```python
from build123d import *

# Parameters (mm, degrees)
BOSS_EXTRUDE1_DEPTH       = 50.8
SHELL1_T                  = -6.35
FILLET1_R                 = 3.175
CUT_EXTRUDE1_DEPTH        = 2.54
F_2_64_TAPPED_HOLE1_D     = 1.778
F_2_64_TAPPED_HOLE1_DEPTH = 6.35
F_2_64_TAPPED_HOLE1_TIP   = 0.53416509


with BuildPart() as part:
    # Sketch2 → Boss-Extrude1 (new body)
    with BuildSketch(Plane(origin=(0, 0, 0), x_dir=(1, 0, 0), z_dir=(0, 1, 0))):
        with BuildLine():
            Line((0, 0), (139.7, 0))
            Line((139.7, 0), (139.7, 63.5))
            ThreePointArc((139.7, 63.5), (111.582381507, 95.881856359), (70.429678072, 107.95))
            Line((70.429678072, 107.95), (0, 107.95))
            Line((0, 107.95), (0, 0))
        make_face()
    extrude(amount=BOSS_EXTRUDE1_DEPTH)

    # Shell1
    shell1_openings = [part.faces().sort_by_distance(p)[0] for p in [
        (71.269444109, 50.8, -57.911371272),
    ]]
    offset(amount=SHELL1_T, openings=shell1_openings, kind=Kind.INTERSECTION)

    # Fillet1
    fillet1_edges = [part.edges().sort_by_distance(p)[0] for p in [
        (6.35, 28.575, -101.6),
        (6.35, 28.575, -6.35),
        (133.35, 28.575, -6.35),
    ]]
    fillet(fillet1_edges, radius=FILLET1_R)

    # Sketch4 → Cut-Extrude1 (cut)
    with BuildSketch(Plane(origin=(0, 50.8, 0), x_dir=(1, 0, 0), z_dir=(0, 1, 0))):
        with BuildLine():
            Line((2.54, 98.425), (2.54, 9.525))
            ThreePointArc((2.54, 9.525), (4.585859133, 4.585859133), (9.525, 2.54))
            Line((9.525, 2.54), (130.175, 2.54))
            ThreePointArc((130.175, 2.54), (135.114140867, 4.585859133), (137.16, 9.525))
            Line((137.16, 9.525), (137.16, 62.940699502))
            ThreePointArc((137.16, 62.940699502), (109.97894276, 93.892185853), (70.429678072, 105.41))
            Line((70.429678072, 105.41), (9.525, 105.41))
            ThreePointArc((9.525, 105.41), (4.585859133, 103.364140867), (2.54, 98.425))
        make_face()
        with BuildLine():
            Line((9.525, 3.81), (130.175, 3.81))
            ThreePointArc((130.175, 3.81), (134.216115254, 5.483884746), (135.89, 9.525))
            Line((135.89, 9.525), (135.89, 62.657254053))
            ThreePointArc((135.89, 62.657254053), (109.178458563, 92.896088268), (70.429678072, 104.14))
            Line((70.429678072, 104.14), (9.525, 104.14))
            ThreePointArc((9.525, 104.14), (5.483884746, 102.466115254), (3.81, 98.425))
            Line((3.81, 98.425), (3.81, 9.525))
            ThreePointArc((3.81, 9.525), (5.483884746, 5.483884746), (9.525, 3.81))
        make_face(mode=Mode.SUBTRACT)
    extrude(amount=-CUT_EXTRUDE1_DEPTH, mode=Mode.SUBTRACT)

    # #2-64 Tapped Hole1
    with Locations(Plane(origin=(0, 50.8, 0), x_dir=(1, 0, 0), z_dir=(0, 1, 0))):
        with Locations((3.175, 3.175), (3.175, 106.3625), (69.85, 106.3625), (138.1125, 63.5), (138.1125, 3.175)):
            Hole(F_2_64_TAPPED_HOLE1_D / 2, depth=F_2_64_TAPPED_HOLE1_DEPTH)
            with Locations((0, 0, -(F_2_64_TAPPED_HOLE1_DEPTH + F_2_64_TAPPED_HOLE1_TIP / 2))):  # 118° drill point
                Cone(0, F_2_64_TAPPED_HOLE1_D / 2, F_2_64_TAPPED_HOLE1_TIP, mode=Mode.SUBTRACT)


solid = part.part
```
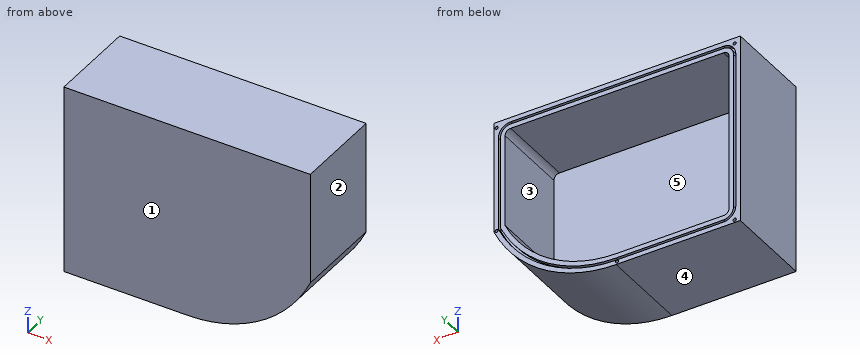
Source: CAD feature listing. Evaluate the final solid. Frame: model axes, mm. Face numbers are marked on the shaded views. A direction names the side the tool comes from. Round coordinates to 2 decimals unless told otherwise and drop trailing zeros. Loops run counter-clockwise (first coordinate to the right, second up) from the corner with the lowest first, then second, coordinate; pieces in that order, holes last. Notation, with made-up numbers: M 42,63.5 L 90,63.5 A20 ccw 90,102.5 Z; hole C 69.25,-35.5 d7. An arc over 180 degrees is marked long. Put each result on its own line as item: value.
(1) Section A-A, the plane y = 18. Return loops of the section in (x, z) (3 decimals), and give its area (3 significant figures).
Solutions:
outline: M 0,-107.95 L 70.43,-107.95 A76.2 ccw 139.7,-63.5 L 139.7,0 L 0,0 Z; hole M 6.35,-98.425 A3.175 ccw 9.525,-101.6 L 70.43,-101.6 A69.85 ccw 133.35,-62.082 L 133.35,-9.525 A3.175 ccw 130.175,-6.35 L 9.525,-6.35 A3.175 ccw 6.35,-9.525 Z
area: 2,830 mm²
(2) Section B-B, the plane z = -58. Return loops of the section in (x, y), and give its area (3 significant figures).
Solutions:
outline: M 0,0 L 139.7,0 L 139.7,50.8 L 137.16,50.8 L 137.16,48.26 L 135.89,48.26 L 135.89,50.8 L 133.35,50.8 L 133.35,6.35 L 6.35,6.35 L 6.35,50.8 L 3.81,50.8 L 3.81,48.26 L 2.54,48.26 L 2.54,50.8 L 0,50.8 Z
area: 1,450 mm²
(3) Pull-direction query (X, two-part tool) for the marked faces 1, 2 and 3; classes: released by +X, released by -X, zero draft, split by the parting line, or undercut.
Solutions:
face 1: zero draft
face 2: released by +X
face 3: undercut
(4) Access query for the marked faces 4 and 5. Directions: +Z, -Z, +X, -X, +Y, -Y. A direction counts if a zero-diameter tool reaches every point of the face in a straight line with its end or side. Return the directions, or none.
Solutions:
face 4: -Z, +X, -X, +Y, -Y
face 5: +Y
(5) First-contact query: pin 1 (1.1 mm diameter, centred on x = 3.18, z = -106.36, fed in from +Y); pin 2 (1.4 mm diameter, centred on x = 138.11, z = -63.5, fed in from +Y); pin 3 (4 mm diameter, centred on x = 85, z = -41.5, fed in from +Y). Flat tips, straight axial feed; report the tip coordinate or a pass-through.
Solutions:
pin 1: y = 44.25
pin 2: y = 44.34
pin 3: y = 6.35
(6) Section C-C, the plane x = 26.5. Return loops of the section in (y, z).
Solutions:
outline: M 0,-107.95 L 50.8,-107.95 L 50.8,-105.41 L 48.26,-105.41 L 48.26,-104.14 L 50.8,-104.14 L 50.8,-101.6 L 6.35,-101.6 L 6.35,-6.35 L 50.8,-6.35 L 50.8,-3.81 L 48.26,-3.81 L 48.26,-2.54 L 50.8,-2.54 L 50.8,0 L 0,0 Z
(7) Ray query, line 1 (Z direction, x = 66.5, y = 38); line 2 (X direction, y = 13, z = -29.5); line 3 (X direction, y = 49.75, z = -63.5). Return the intervals inside material, ascending. Write a range as [from, to].
Solutions:
line 1: [-107.95, -101.6], [-6.35, 0]
line 2: [0, 6.35], [133.35, 139.7]
line 3: [0, 2.54], [3.81, 6.35], [132.65, 135.49], [136.9, 137.22], [139, 139.7]
